Here's how the part is built. I have some questions about the finished solid (model axes, mm). Face numbers are marked on the shaded views. Round coordinates to 2 decimals unless told otherwise and drop trailing zeros. Loops run counter-clockwise (first coordinate to the right, second up) from the corner with the lowest first, then second, coordinate; pieces in that order, holes last. Notation, with made-up numbers: M 87.5,-11.5 L 133.5,-11.5 A21 cw 133.5,19.5 Z; hole C 21,18 d2. An arc over 180 degrees is marked long. Answer as a JSON object with one key per item and string values.
from build123d import *

# Parameters (mm, degrees)
F0_W      = 1000
F0_H      = 1000
F1_DEPTH  = 100
F3_DEPTH  = 20
F4_SIZE   = 9.99999
F5_W      = 50
F5_H      = 50
F6_DEPTH  = 1000
F7_W      = 61.6666623382
F7_H      = 50
F8_DEPTH  = 1000
F9_W      = 1000
F9_H      = 1000
F9_W_2    = 50
F9_H_2    = 50
F9_W_3    = 61.6666623382
F10_W     = 57.3770701885
F10_H     = 57.3770701885
F10_W_2   = 65.0272965431
F10_H_2   = 76.5027403831
F11_DEPTH = 7
F12_W     = 66.2613213062
F12_H     = 68.3319568634
F13_DEPTH = 1000
F14_W     = 65.0273263454
F14_H     = 70.7650482655
F15_DEPTH = 1000


# Not quite as in the source:
# - a fillet or chamfer is up to 0.001 mm smaller than in the source, because OpenCascade refuses the exact size


with BuildPart() as f1:
    # F0 (on Top) → F1 (new body)
    with BuildSketch(Plane.XY):
        Rectangle(F0_W, F0_H)
    extrude(amount=F1_DEPTH)

    # F2 (on face) → F3 (cut)
    with BuildSketch(Plane.XY.offset(100)):
        Polygon((72.4873734153, -175), (175, -72.4873734153), (175, 72.4873734153), (72.4873734153, 175), (-72.4873734153, 175), (-175, 72.4873734153), (-175, -72.4873734153), (-72.4873734153, -175), align=None)
    extrude(amount=-F3_DEPTH, mode=Mode.SUBTRACT)

    # F4 (size 10 in the source; OpenCascade refuses exactly that, so slightly less here)
    f4_edges = [f1.edges().sort_by_distance(p)[0] for p in [
        (123.743687, -123.743687, 80),
        (175, 0, 80),
        (123.743687, 123.743687, 80),
        (0, 175, 80),
        (-123.743687, 123.743687, 80),
        (-175, 0, 80),
        (-123.743687, -123.743687, 80),
        (0, -175, 80),
        (0, -500, 100),
        (-500, 0, 100),
        (500, 0, 100),
        (0, 500, 100),
        (123.743687, -123.743687, 100),
        (175, 0, 100),
        (123.743687, 123.743687, 100),
        (0, 175, 100),
        (-123.743687, 123.743687, 100),
        (-175, 0, 100),
        (-123.743687, -123.743687, 100),
        (0, -175, 100),
    ]]
    chamfer(f4_edges, length=F4_SIZE)

    # F5 (on face) → F6 (join)
    with BuildSketch(Plane(origin=(0, 0, 0), x_dir=(1, 0, 0), z_dir=(0, 0, -1))):
        with Locations((-425, 425)):
            Rectangle(F5_W, F5_H)
    extrude(amount=F6_DEPTH)

    # F7 (on face) → F8 (join)
    with BuildSketch(Plane(origin=(0, 0, 0), x_dir=(1, 0, 0), z_dir=(0, 0, -1))):
        with Locations((412.1584743261, 433.19670856)):
            Rectangle(F7_W, F7_H)
    extrude(amount=F8_DEPTH)

    # F9 (on face) + F10 (on face) → F11 (join)
    with BuildSketch(Plane(origin=(0, 0, 0), x_dir=(1, 0, 0), z_dir=(0, 0, -1))):
        Rectangle(F9_W, F9_H)
        with Locations((-425, 425)):
            Rectangle(F9_W_2, F9_H_2, mode=Mode.SUBTRACT)
        with Locations((412.1584743261, 433.19670856)):
            Rectangle(F9_W_3, F9_H_2, mode=Mode.SUBTRACT)
    with BuildSketch(Plane(origin=(0, 0, 0), x_dir=(1, 0, 0), z_dir=(0, 0, -1))):
        with Locations((-409.2896133661, -459.9726945162)):
            Rectangle(F10_W, F10_H)
        with Locations((434.1530203819, -438.9344155788)):
            Rectangle(F10_W_2, F10_H_2)
    extrude(amount=F11_DEPTH)

    # F12 (on face) → F13 (join)
    with BuildSketch(Plane(origin=(0, 0, -7), x_dir=(1, 0, 0), z_dir=(0, 0, -1))):
        with Locations((-417.2714799643, -440.7140314579)):
            Rectangle(F12_W, F12_H)
    extrude(amount=F13_DEPTH)

    # F14 (on face) → F15 (join)
    with BuildSketch(Plane(origin=(0, 0, -7), x_dir=(1, 0, 0), z_dir=(0, 0, -1))):
        with Locations((447.5409835577, -443.7158554792)):
            Rectangle(F14_W, F14_H)
    extrude(amount=F15_DEPTH)


solid = f1.part
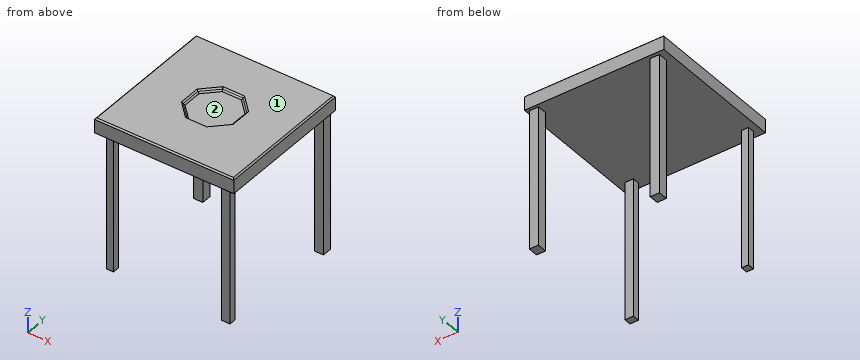
Item 1: I want a section at D-D, the plane y = 282. Please give me the cut outline in (x, z), then the cut area to 3 significant figures.
Resolved:
{"outline": "M -500,-7 L 500,-7 L 500,90 L 490,100 L -490,100 L -500,90 Z", "area": "107,000 mm²"}
Item 2: I want a section at A-A, the plane z = -504. Please give me the cut outline in (x, y), then the cut area to 3 significant figures.
Resolved:
{"outline": "M -450.4,406.55 L -384.14,406.55 L -384.14,474.88 L -450.4,474.88 Z; M -450,-450 L -400,-450 L -400,-400 L -450,-400 Z; M 381.33,-458.2 L 442.99,-458.2 L 442.99,-408.2 L 381.33,-408.2 Z; M 415.03,408.33 L 480.05,408.33 L 480.05,479.1 L 415.03,479.1 Z", "area": "14,700 mm²"}
Item 3: I'm going to push flat-ended pins straight in: pin 1 Ø3 at (x, y) = (-217, -394) entering from -Z; pin 2 Ø20.5 at (y, z) = (439.5, -715) entering from +X; pin 3 Ø20 at (x, z) = (-407, -692.5) entering from -Y. Where does each tip first touch, or does it pass through?
Resolved:
{"pin 1": "z = -7", "pin 2": "x = 480.05", "pin 3": "y = -450"}
Item 4: Please list where these lines run through material, in increasing order: probe 1 along Y at (x, z) = (-447.5, -532); probe 2 along Z at (x, y) = (-366, 252); probe 3 along Y at (x, z) = (410.5, -52). Write a range as from..to.
Resolved:
{"probe 1": "-450..-400, 406.55..474.88", "probe 2": "-7..100", "probe 3": "-458.2..-408.2"}
Item 5: If we mould it in two halves opening along X, with no side actions, what happens to the marked faces 1 and 2? For each: pulls with the +X half, pulls with the -X half, needs draft (parallel to the pull), parting line crosses it, or undercut.
Resolved:
{"face 1": "needs draft", "face 2": "undercut"}
